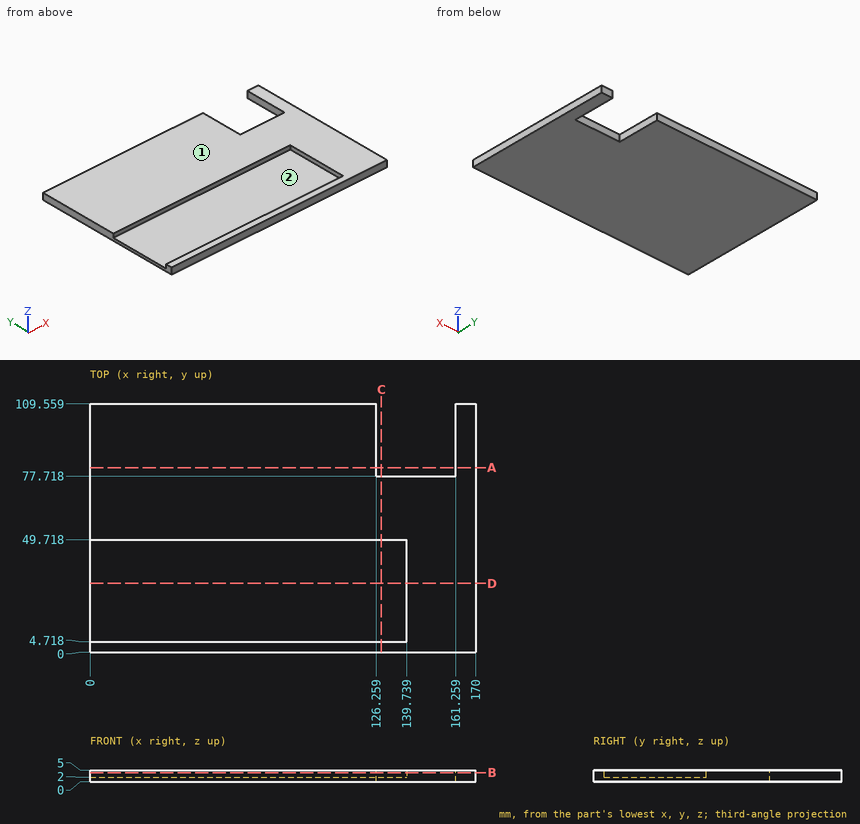
Verification items for this drawing (mm, ordinates from the low corner). Coordinates: 2 decimals unless noted, no trailing zeros. Order: outer loops, then holes, each group sorted by start corner. A loop starts at its lowest first (then second) coordinate and runs counter-clockwise, first axis right, second up. Notation, with made-up numbers: M -26.5,-9 L 3.5,-9 A14 ccw 3.5,17 Z; hole C -11,52 d2. An arc over 180 degrees is marked long. Use CSV: the item, a comma, the result in double quotes.
Item 1: Mould release check, pull along Y, two halves, no side actions. Record for the marked faces 1 and 2: pulls with the +Y half, pulls with the -Y half, needs draft (parallel to the pull), parting line crosses it, or undercut.
Returned:
face 1,"needs draft"
face 2,"undercut"
Item 2: Cross-section at D-D on y = 30.5. Record the cut outline in (x, z).
Returned:
outline,"M 0,0 L 170,0 L 170,5 L 139.74,5 L 139.74,2 L 0,2 Z"
Item 3: Cross-section at A-A on y = 81.5. Record the cut outline in (x, z), then the cut area to 3 significant figures.
Returned:
outline,"M 0,0 L 126.26,0 L 126.26,5 L 0,5 Z; M 161.26,0 L 170,0 L 170,5 L 161.26,5 Z"
area,"675 mm2"
Item 4: Thickness scan on line 1 along Y through (x, z) = (11.5, 3.4); line 2 along X through (y, z) = (101, 0.85); line 3 along Y through (x, z) = (133, 2.1). Record the ranges inside material, lowest first.
Returned:
line 1,"y = 0 to 4.72, 49.72 to 109.56"
line 2,"x = 0 to 126.26, 161.26 to 170"
line 3,"y = 0 to 4.72, 49.72 to 77.72"
Item 5: Cross-section at B-B on z = 4.1. Record the cut outline in (x, y), then the cut area to 3 significant figures.
Returned:
outline,"M 0,0 L 170,0 L 170,109.56 L 161.26,109.56 L 161.26,77.72 L 126.26,77.72 L 126.26,109.56 L 0,109.56 L 0,49.72 L 139.74,49.72 L 139.74,4.72 L 0,4.72 Z"
area,"11,200 mm2"
Item 6: Cross-section at C-C on x = 128.5. Record the cut outline in (y, z).
Returned:
outline,"M 0,0 L 77.72,0 L 77.72,5 L 49.72,5 L 49.72,2 L 4.72,2 L 4.72,5 L 0,5 Z"
Item 7: Gauge pin test, flat ends, axial feed: pin 1 Ø6 at (x, y) = (43, 40) entering from +Z; pin 2 Ø2.5 at (y, z) = (31.5, 3.5) entering from -X. Record the tip position at first contact, or that the pin passes through.
Returned:
pin 1,"stops at z = 2"
pin 2,"stops at x = 139.74"
